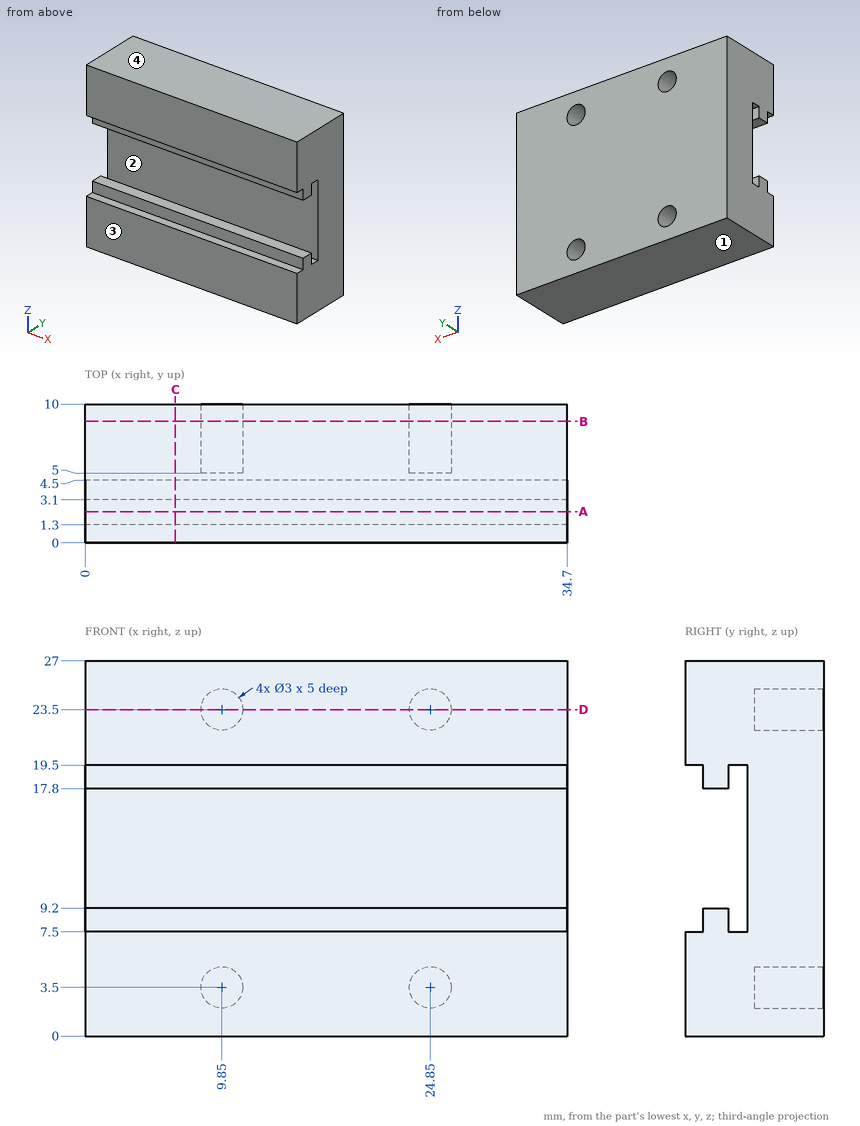
Source: three-view drawing plus pictorial views. Frame: mm from the lowest corner of the part. Coordinates: 2 decimals unless noted, no trailing zeros. Loops run counter-clockwise (first coordinate to the right, second up) from the corner with the lowest first, then second, coordinate; pieces in that order, holes last. Notation, with made-up numbers: (76, -21) - (108, -21) arc R23 cw to (108, 13) - close; hole circle Ø9 at (2.5, -3.5). An arc over 180 degrees is marked (long way). One line per item, written item: value. Start each with the question number.
1. Section B-B (y = 8.75). Return the cut outline in (x, z).
2. Section A-A (y = 2.25). Return the cut outline in (x, z), and give its area (3 significant figures).
3. Contact query for flat-ended pins moving along their axis: P1, Ø1.4, axis at x = 15, z = 8.5, coming from the -Y side; P2, Ø0.9, axis at x = 24.5, z = 23, coming from the +Y side. Output: stop coordinate, or through.
4. Ray query, L1, parallel to X at y = 7.05, z = 23.5; L2, parallel to Z at x = 9.85, y = 9.05; L3, parallel to Z at x = 13, y = 1.25. Return the intervals inside material, ascending.
5. Section C-C (x = 6.5). Return the cut outline in (y, z).
6. Section D-D (z = 23.5). Return the cut outline in (x, y).
7. Mould query, pull axis Z, two halves, no side actions, for the marked faces 1, 2, 3 and 4. Classes: pulls with the +Z half, pulls with the -Z half, needs draft (parallel to the pull), parting line crosses it, or undercut.
Verdict:
1. outline: (0, 0) - (34.7, 0) - (34.7, 27) - (0, 27) - close; hole circle Ø3 at (9.85, 3.5); hole circle Ø3 at (9.85, 23.5); hole circle Ø3 at (24.85, 3.5); hole circle Ø3 at (24.85, 23.5)
2. outline: (0, 0) - (34.7, 0) - (34.7, 9.2) - (0, 9.2) - close; (0, 17.8) - (34.7, 17.8) - (34.7, 27) - (0, 27) - close
2. area: 638 mm2
3. P1: stops at y = 1.3
3. P2: stops at y = 5
4. L1: x = 0 to 8.35, 11.35 to 23.35, 26.35 to 34.7
4. L2: z = 0 to 2, 5 to 22, 25 to 27
4. L3: z = 0 to 7.5, 19.5 to 27
5. outline: (0, 0) - (10, 0) - (10, 27) - (0, 27) - (0, 19.5) - (1.3, 19.5) - (1.3, 17.8) - (3.1, 17.8) - (3.1, 19.5) - (4.5, 19.5) - (4.5, 7.5) - (3.1, 7.5) - (3.1, 9.2) - (1.3, 9.2) - (1.3, 7.5) - (0, 7.5) - close
6. outline: (0, 0) - (34.7, 0) - (34.7, 10) - (26.35, 10) - (26.35, 5) - (23.35, 5) - (23.35, 10) - (11.35, 10) - (11.35, 5) - (8.35, 5) - (8.35, 10) - (0, 10) - close
7. face 1: pulls with the -Z half
7. face 2: undercut
7. face 3: needs draft
7. face 4: pulls with the +Z half
